Can you work these out from the drawing? Everything is in mm from the part's minimum corner. A direction names the side the tool comes from. Coordinates: 2 decimals unless noted, no trailing zeros. Write each loop counter-clockwise with the first axis right and the second up, starting at its lowest first coordinate (ties: lowest second). Pieces come first, ordered by that corner, then holes. Notation, with made-up numbers: M -12.5,-2 L 10.5,-2 A32 cw 10.5,24 Z; hole C 40.25,32 d11. An arc over 180 degrees is marked long. Write each question's results on one line, items separated by ' | '. Start each with the question number.
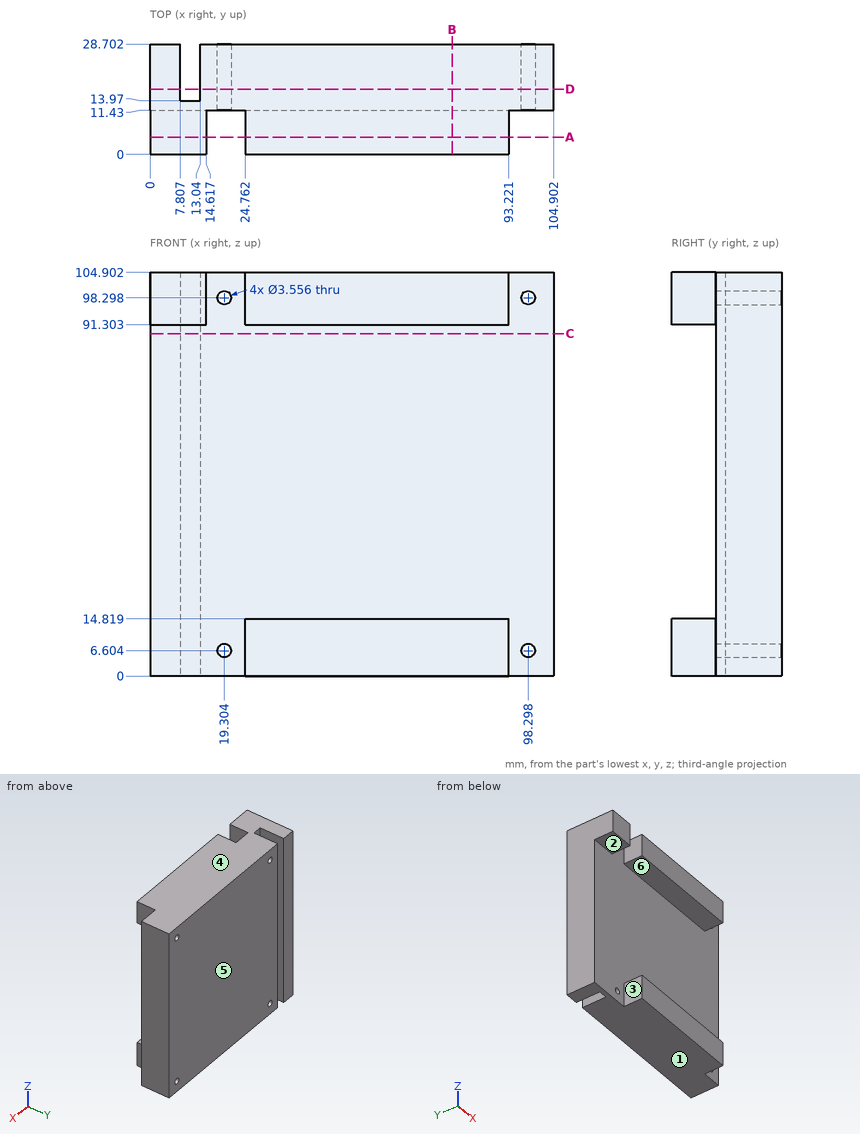
1) I want a section at C-C, the plane z = 89. Write out the boundary of the cut face in (x, y), then the cut area to 3 significant figures.
2) Please list where these lines run through material, in increasing order: line 1 (Z direction, x = 68.5, y = 3); line 2 (X direction, y = 7.5, z = 100); line 3 (X direction, y = 18.25, z = 22.5). Write a range as [from, to].
3) I want a section at D-D, the plane y = 17. Write out the boundary of the cut face in (x, z), then the cut area to 3 significant figures.
4) We'd pull the mould along Z, two halves only. Please class the marked faces 4, 5 and 6: pulls with the +Z half, pulls with the -Z half, needs draft (parallel to the pull), parting line crosses it, or undercut.
5) I want a section at B-B, the plane x = 78.5. Write out the boundary of the cut face in (y, z), then the cut area to 3 significant figures.
6) For pin 1 Ø3 at (y, z) = (10.5, 85.5) entering from +X; pin 2 Ø5.5 at (y, z) = (7.5, 11) entering from -X; pin 3 Ø3 at (x, z) = (98.298, 98.298) entering from -Y; pin 4 Ø3.5 at (y, z) = (4.5, 100) entering from +X, each with a flat end and sliding along its axis, tell me the tip position at first contact or that it passes through.
7) I want a section at A-A, the plane y = 4.5. Write out the boundary of the cut face in (x, z).
8) For the marked faces 1, 2 and 3, which set-ups out of +Z, -Z, +X, -X, +Y, -Y let a thin tool reach every point of the face, with its end or its side?
Output:
1) outline: M 0,11.43 L 104.9,11.43 L 104.9,28.7 L 13.04,28.7 L 13.04,13.97 L 7.81,13.97 L 7.81,28.7 L 0,28.7 Z | area: 1,730 mm2
2) line 1: z = [0, 14.82], [91.3, 104.9] | line 2: x = [0, 14.62], [24.76, 93.22] | line 3: x = [0, 7.81], [13.04, 104.9]
3) outline: M 0,0 L 7.81,0 L 7.81,104.9 L 0,104.9 Z; M 13.04,0 L 104.9,0 L 104.9,104.9 L 13.04,104.9 Z; hole C 19.3,6.6 d3.56; hole C 19.3,98.3 d3.56; hole C 98.3,6.6 d3.56; hole C 98.3,98.3 d3.56 | area: 10,400 mm2
4) face 4: pulls with the +Z half | face 5: needs draft | face 6: undercut
5) outline: M 0,0 L 28.7,0 L 28.7,104.9 L 0,104.9 L 0,91.3 L 11.43,91.3 L 11.43,14.82 L 0,14.82 Z | area: 2,140 mm2
6) pin 1: stops at x = 104.9 | pin 2: stops at x = 24.76 | pin 3: passes through | pin 4: stops at x = 93.22
7) outline: M 0,91.3 L 14.62,91.3 L 14.62,104.9 L 0,104.9 Z; M 24.76,0 L 93.22,0 L 93.22,14.82 L 24.76,14.82 Z; M 24.76,91.3 L 93.22,91.3 L 93.22,104.9 L 24.76,104.9 Z
8) face 1: -Z, +X, -X, +Y, -Y | face 2: -Z, +X, -X, -Y | face 3: +Z, -Z, -X, -Y
